Design review of the part built by this model. Coordinates are the model's own, in mm. Face numbers are marked on the shaded views. A direction names the side the tool comes from. Round coordinates to 2 decimals unless told otherwise and drop trailing zeros. Write each loop counter-clockwise with the first axis right and the second up, starting at its lowest first coordinate (ties: lowest second). Pieces come first, ordered by that corner, then holes. Notation, with made-up numbers: (-16.5, -11.5) -> (33.5, -11.5) arc R19 cw to (33.5, 20.5) -> close; hole circle Ø2 at (67.25, -38). An arc over 180 degrees is marked (long way). One line per question, with ' | ' between items. Start each with the question number.
1) Consider section A-A (x = -4). Give the boundary of the cut face in (y, z), then the cut area to 3 significant figures.
2) For the marked faces 4, 5, 6 and 7, list the 3-axis set-ups (+Z, -Z, +X, -X, +Y, -Y) from which the entire face can be reached by the end or side of a thin tool; tool diameter is ignored.
3) Mouldability with a two-part tool opening along X and no side actions: class the marked faces 1, 2 and 3 as +X half, -X half, draft (parallel to the pull), parting line (faces both ways), or undercut.
4) Consider section B-B (z = 5). Give the boundary of the cut face in (x, y), then the cut area to 3 significant figures.
5) For probe 1 along Y at (x, z) = (0, 6.5); probe 2 along X at (y, z) = (-13.5, 4.5); probe 3 along Y at (x, z) = (-13, 2.75), list the stretches that pass through material, from the lowest coordinate up.
6) Insertion check: pin 1 Ø2 at (x, z) = (22, 8) entering from -Y; pin 2 Ø3 at (y, z) = (-9.5, 2.5) entering from -X; pin 3 Ø4 at (y, z) = (20, 9) entering from +X. Each pin has a flat end and moves straight along its axis. Give the tip position at first contact, or say it passes through.
7) Consider section C-C (y = 0). Give the boundary of the cut face in (x, z), then the cut area to 3 significant figures.
8) Consider section D-D (z = 10). Give the boundary of the cut face in (x, y).
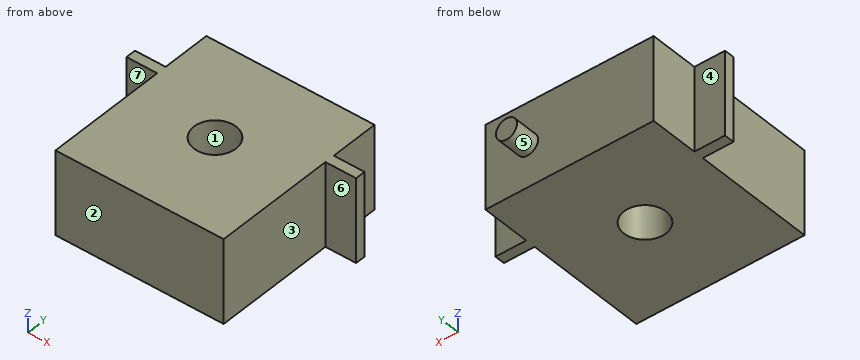
```python
from build123d import *

# Parameters (mm, degrees)
SKETCH1_W           = 40
SKETCH1_H           = 43
SKETCH1_R           = 5
BOSS_EXTRUDE1_DEPTH = 20
SKETCH2_R           = 2.5
BOSS_EXTRUDE2_DEPTH = 6
SKETCH3_W           = 20
SKETCH3_H           = 2.4
BOSS_EXTRUDE3_DEPTH = 7.3


with BuildPart() as part:
    # Sketch1 → Boss-Extrude1 (new body)
    with BuildSketch(Plane.XY):
        Rectangle(SKETCH1_W, SKETCH1_H)
        Circle(SKETCH1_R, mode=Mode.SUBTRACT)
    extrude(amount=BOSS_EXTRUDE1_DEPTH)

    # Sketch2 → Boss-Extrude2 (add)
    with BuildSketch(Plane(origin=(0, 21.5, 0), x_dir=(1, 0, 0), z_dir=(0, 1, 0))):
        with Locations((10, -10)):
            Circle(SKETCH2_R)
    extrude(amount=BOSS_EXTRUDE2_DEPTH)

    # Sketch3 → Boss-Extrude3 (add)
    with BuildSketch(Plane.ZY.offset(20)):
        with Locations((10, 8.7)):
            Rectangle(SKETCH3_W, SKETCH3_H)
    boss_extrude3 = extrude(amount=BOSS_EXTRUDE3_DEPTH)

    # Mirror1: Boss-Extrude3 across plane
    add(boss_extrude3.mirror(Plane(origin=(0, 0, 0), x_dir=(0, 0, 1), z_dir=(1, 0, 0))))


solid = part.part
```
From the geometry:
1) outline: (-21.5, 0) -> (-3, 0) -> (-3, 20) -> (-21.5, 20) -> close; (3, 0) -> (21.5, 0) -> (21.5, 20) -> (3, 20) -> close | area: 740 mm2
2) face 4: +Z, -Z, -X, +Y | face 5: +Y | face 6: +Z, -Z, +X, -Y | face 7: +Z, -Z, -X, -Y
3) face 1: undercut | face 2: draft | face 3: +X half
4) outline: (-27.3, 7.5) -> (-20, 7.5) -> (-20, -21.5) -> (20, -21.5) -> (20, 7.5) -> (27.3, 7.5) -> (27.3, 9.9) -> (20, 9.9) -> (20, 21.5) -> (-20, 21.5) -> (-20, 9.9) -> (-27.3, 9.9) -> close; hole circle Ø10 at (0, 0) | area: 1,680 mm2
5) probe 1: y = -21.5 to -5, 5 to 21.5 | probe 2: x = -20 to 20 | probe 3: y = -21.5 to 21.5
6) pin 1: stops at y = 7.5 | pin 2: stops at x = -20 | pin 3: stops at x = 20
7) outline: (-20, 0) -> (-5, 0) -> (-5, 20) -> (-20, 20) -> close; (5, 0) -> (20, 0) -> (20, 20) -> (5, 20) -> close | area: 600 mm2
8) outline: (-27.3, 7.5) -> (-20, 7.5) -> (-20, -21.5) -> (20, -21.5) -> (20, 7.5) -> (27.3, 7.5) -> (27.3, 9.9) -> (20, 9.9) -> (20, 21.5) -> (12.5, 21.5) -> (12.5, 27.5) -> (7.5, 27.5) -> (7.5, 21.5) -> (-20, 21.5) -> (-20, 9.9) -> (-27.3, 9.9) -> close; hole circle Ø10 at (0, 0)
